Input: dimensioned drawing with shaded views. Units: mm. Origin: part minimum x, y, z. Give positions to 0.01 mm unless a question says otherwise; leave off trailing zeros. Write each loop counter-clockwise with the first axis right and the second up, starting at its lowest first coordinate (ties: lowest second). Pieces come first, ordered by that corner, then holes.
Q1. Section C-C (z = 28). Return the cut outline in (x, y), plus the area to 3 significant figures.
Q2. Line query: line 1 (Y direction, x = 7.5, z = 75.5); line 2 (Y direction, x = 7, z = 56.5); line 3 (Y direction, x = 5.5, z = 71). Output: solid intervals per line, ascending.
Q3. Pin query (flat end, axial travel): pin 1 Ø1 at (y, z) = (13, 28) entering from +X; pin 2 Ø2 at (y, z) = (3, 61) entering from +X; pin 3 Ø1 at (y, z) = (5, 54) entering from -X. Return the tip coordinate at first contact, or that it passes through.
Q4. Section D-D (y = 2.75). Return the cut outline in (x, z).
Q5. Section A-A (z = 8.5). Return the cut outline in (x, y), plus the area to 3 significant figures.
Q6. Section B-B (x = 1.5). Return the cut outline in (y, z).
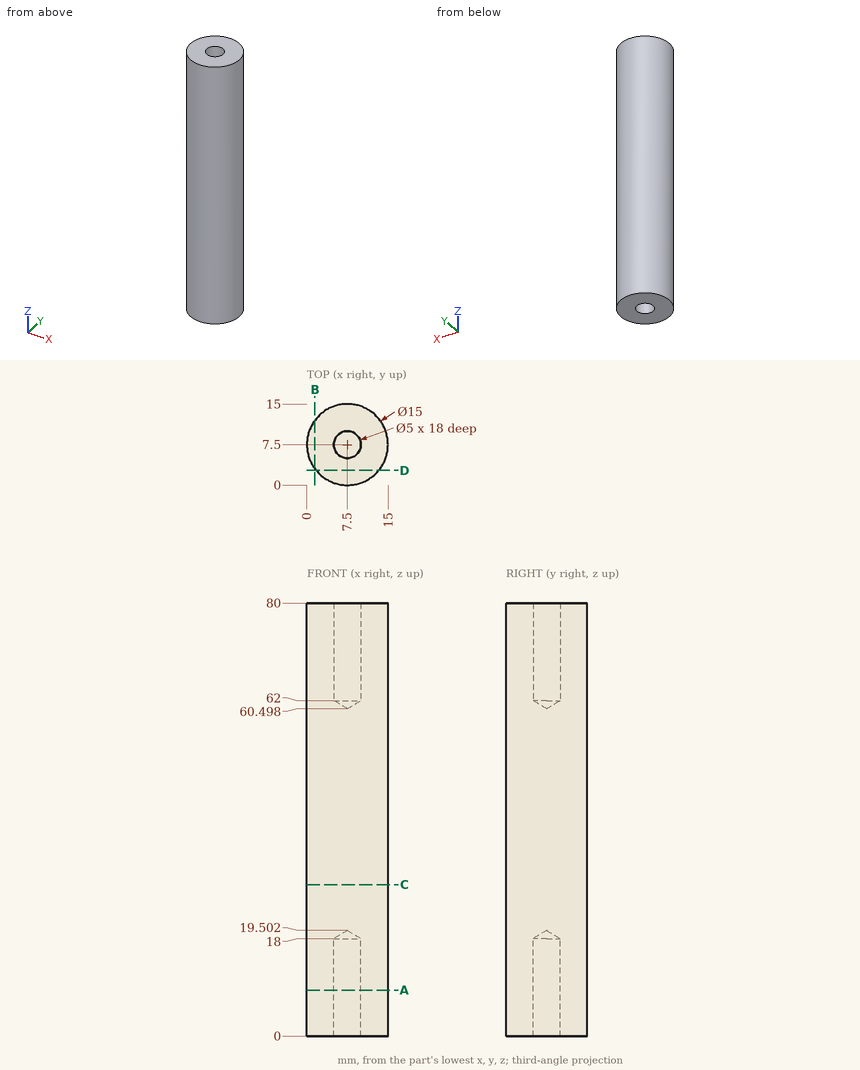
Computed:
1. outline: circle Ø15 at (7.5, 7.5)
1. area: 177 mm2
2. line 1: y = 0 to 5, 10 to 15
2. line 2: y = 0.02 to 14.98
2. line 3: y = 0.27 to 6, 9 to 14.73
3. pin 1: stops at x = 13.09
3. pin 2: stops at x = 14.13
3. pin 3: stops at x = 0.27
4. outline: (1.7, 0) - (13.3, 0) - (13.3, 80) - (1.7, 80) - close
5. outline: circle Ø15 at (7.5, 7.5); hole circle Ø5 at (7.5, 7.5)
5. area: 157 mm2
6. outline: (3, 0) - (12, 0) - (12, 80) - (3, 80) - close
